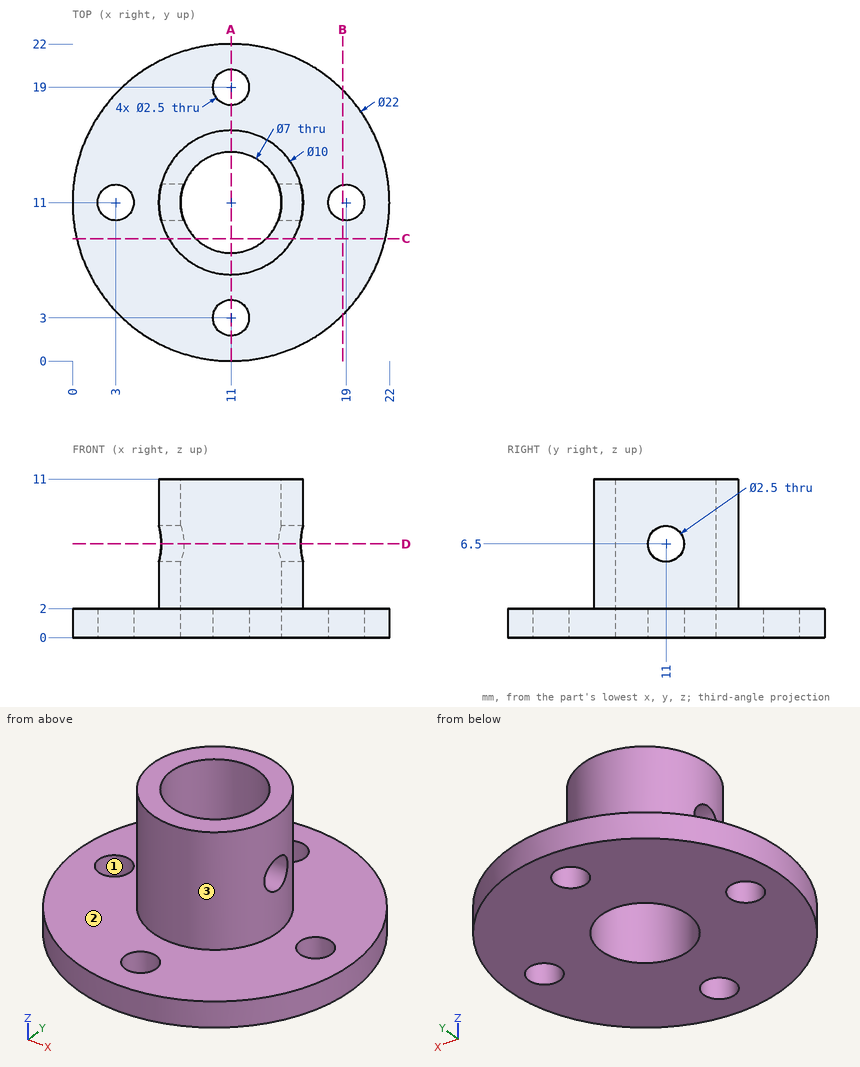
Answer from the drawing. Dimensions are ordinates in mm from the lowest x, y and z of the part. Round coordinates to 2 decimals unless told otherwise and drop trailing zeros. Write each loop counter-clockwise with the first axis right and the second up, starting at its lowest first coordinate (ties: lowest second). Pieces come first, ordered by that corner, then holes. Notation, with made-up numbers: M 56.25,-25 L 76.25,-25 A28 ccw 76.25,6 Z; hole C 0.5,69.25 d3. An arc over 180 degrees is marked long. Write each question's results on one line, items separated by ' | '. Start each with the question number.
Item 1: Flat-ended cylindrical pins translate along their axes: pin 1 Ø2 at (x, y) = (10.5, 17.5) entering from +Z; pin 2 Ø3 at (y, z) = (11, 6.5) entering from +X; pin 3 Ø3 at (x, z) = (13.5, 3) entering from -Y. Find the tip coordinate at first contact, or state that the pin passes through.
Item 2: Straight lines are drawn through the part: L1, parallel to Y at x = 11, z = 0.7; L2, parallel to Z at x = 3.5, y = 8.5; L3, parallel to X at y = 8.25, z = 8.5. For each, find the intervals that lie inside material, in ascending order. Write a range as [from, to].
Item 3: A cutting plane is placed at B-B on x = 18.75. Write down the section's boundary in (y, z).
Item 4: A cutting plane is placed at A-A on x = 11. Write down the section's boundary in (y, z).
Item 5: For a pull along X with two mould halves and no side action, classify the marked faces 1, 2 and 3 as pulls with the +X half, pulls with the -X half, needs draft (parallel to the pull), parting line crosses it, or undercut.
Item 6: A cutting plane is placed at C-C on y = 8.5. Write down the section's boundary in (x, z).
Item 7: A cutting plane is placed at D-D on z = 6.5. Write down the section's boundary in (x, y), and give its area (3 significant figures).
Check sheet entries:
1) pin 1: z = 2 | pin 2: x = 16 | pin 3: y = 0.09
2) L1: [0, 1.75], [4.25, 7.5], [14.5, 17.75], [20.25, 22] | L2: [0, 2] | L3: [6.82, 8.83], [13.17, 15.18]
3) outline: M 3.19,0 L 9.78,0 L 9.78,2 L 3.19,2 Z; M 12.22,0 L 18.81,0 L 18.81,2 L 12.22,2 Z
4) outline: M 0,0 L 1.75,0 L 1.75,2 L 0,2 Z; M 4.25,0 L 7.5,0 L 7.5,11 L 6,11 L 6,2 L 4.25,2 Z; M 14.5,0 L 17.75,0 L 17.75,2 L 16,2 L 16,11 L 14.5,11 Z; M 20.25,0 L 22,0 L 22,2 L 20.25,2 Z
5) face 1: undercut | face 2: needs draft | face 3: parting line crosses it
6) outline: M 0.29,0 L 8.55,0 L 8.55,11 L 6.67,11 L 6.67,2 L 0.29,2 Z; M 13.45,0 L 21.71,0 L 21.71,2 L 15.33,2 L 15.33,11 L 13.45,11 Z
7) outline: M 6.16,9.75 A5 ccw 15.84,9.75 L 14.27,9.75 A3.5 cw 7.73,9.75 Z; M 6.16,12.25 L 7.73,12.25 A3.5 cw 14.27,12.25 L 15.84,12.25 A5 ccw Z | area: 32.4 mm²
